from build123d import *

# Parameters (mm, degrees)
F0_R     = 5.5
F0_R_2   = 1
F1_DEPTH = 3
F2_R     = 5
F2_R_2   = 1
F3_DEPTH = 3
F4_W     = 8
F4_H     = 6
F4_R     = 1
F5_DEPTH = 8
F6_R     = 1
F7_DEPTH = 25


with BuildPart() as f1:
    # F0 (on Top) → F1 (new body)
    with BuildSketch(Plane.XY):
        with Locations((-27.4031814188, 27.8583839536)):
            Circle(F0_R)
        with Locations((-27.4031814188, 27.8583839536)):
            Circle(F0_R_2, mode=Mode.SUBTRACT)
    extrude(amount=F1_DEPTH)

    # F2 (on face) → F3 (join)
    with BuildSketch(Plane.XY.offset(3)):
        with Locations((-27.4031814188, 27.8583839536)):
            Circle(F2_R)
        with Locations((-27.4031814188, 27.8583839536)):
            Circle(F2_R_2, mode=Mode.SUBTRACT)
    extrude(amount=F3_DEPTH)

    # F4 (on face) → F5 (join)
    with BuildSketch(Plane.XY.offset(6)):
        with Locations((-27.4031814188, 27.8583839536)):
            Rectangle(F4_W, F4_H)
        with Locations((-27.4031814188, 27.8583839536)):
            Circle(F4_R, mode=Mode.SUBTRACT)
        with Locations((-27.4031814188, 27.8583839536)):
            Circle(F4_R)
    extrude(amount=F5_DEPTH)

    # F6 (on face) → F7 (cut)
    with BuildSketch(Plane.XZ.offset(-24.8583839536)):
        with Locations((-27.4031814188, 10)):
            Circle(F6_R)
    extrude(amount=-F7_DEPTH, mode=Mode.SUBTRACT)


solid = f1.part
Check sheet for the modelled part. Datum: model origin and axes. Units: mm. A direction names the side the tool comes from. Give positions to 0.01 mm unless a question says otherwise; leave off trailing zeros. Write each loop counter-clockwise with the first axis right and the second up, starting at its lowest first coordinate (ties: lowest second). Pieces come first, ordered by that corner, then holes. Notation, with made-up numbers: (69.25, 1.25) -> (73.25, 1.25) arc R32 cw to (73.25, 33.25) -> close; hole circle Ø10 at (-21.5, -2). An arc over 180 degrees is marked (long way). Write item = value, one per line.
Item 1: Gauge pin test, flat ends, axial feed: pin 1 (2 mm diameter, centred on x = -28.5, y = 32, fed in from +Z); pin 2 (3 mm diameter, centred on y = 25, z = 9.5, fed in from -X); pin 3 (0.6 mm diameter, centred on x = -27, y = 27.5, fed in from -Z); pin 4 (4 mm diameter, centred on x = -28.5, y = 26.5, fed in from -Z). Record the tip position at first contact, or that the pin passes through.
Output:
pin_1 = 6
pin_2 = -31.4
pin_3 = 6
pin_4 = 0
Item 2: Sectioned sample at B-B on x = -27.5. Record the boundary of the cut face in (y, z).
Output:
outline = (22.36, 0) -> (26.86, 0) -> (26.86, 6) -> (28.85, 6) -> (28.85, 0) -> (33.36, 0) -> (33.36, 3) -> (32.86, 3) -> (32.86, 6) -> (30.86, 6) -> (30.86, 9) -> (24.86, 9) -> (24.86, 6) -> (22.86, 6) -> (22.86, 3) -> (22.36, 3) -> close; (24.86, 11) -> (30.86, 11) -> (30.86, 14) -> (24.86, 14) -> close
Item 3: Sectioned sample at C-C on y = 28.25. Record the boundary of the cut face in (x, z), and give its area (3 significant figures).
Output:
outline = (-32.89, 0) -> (-28.32, 0) -> (-28.32, 6) -> (-26.48, 6) -> (-26.48, 0) -> (-21.92, 0) -> (-21.92, 3) -> (-22.42, 3) -> (-22.42, 6) -> (-23.4, 6) -> (-23.4, 14) -> (-31.4, 14) -> (-31.4, 6) -> (-32.39, 6) -> (-32.39, 3) -> (-32.89, 3) -> close; hole circle Ø2 at (-27.4, 10)
area = 113 mm^2
Item 4: Sectioned sample at D-D on x = -24.5. Record the boundary of the cut face in (y, z), and give its area (3 significant figures).
Output:
outline = (23.19, 0) -> (32.53, 0) -> (32.53, 3) -> (31.93, 3) -> (31.93, 6) -> (30.86, 6) -> (30.86, 14) -> (24.86, 14) -> (24.86, 6) -> (23.79, 6) -> (23.79, 3) -> (23.19, 3) -> close
area = 100 mm^2
Item 5: Scan lines: probe 1 along Z at (x, y) = (-27.75, 31); probe 2 along X at (y, z) = (28.75, 11.5); probe 3 along Y at (x, z) = (-28, 7). Record each from-to range of solid material in increasing order. Write a range as from..to.
Output:
probe_1 = 0..6
probe_2 = -31.4..-23.4
probe_3 = 24.86..30.86
Item 6: Tool access check on faces 4 (the flat face through (-27, 24, 6)), 5 (the flat face through (-26.6, 30.858, 9.1)), 6 (the cylindrical face through (-31.088, 31.238, 4.479)), 7 (the flat face through (-27, 28, 6)). Record the directions out of +Z, -Z, +X, -X, +Y, -Y that give a thin tool (end or side, any length) a straight path to the whole face; none if there is none.
Output:
face_4 = +Z, +X, -X, -Y
face_5 = +Z, +X, -X, +Y
face_6 = +Z
face_7 = -Z
Item 7: Release check for a two-part mould opening along X. For faces 1 (the cylindrical face through (-26.45, 27.82, 10.3)), 2 (the flat face through (-23.403, 28, 10)), 3 (the flat face through (-27, 32, 6)) record: +X half, -X half, draft (parallel to the pull), parting line (faces both ways), or undercut.
Output:
face_1 = undercut
face_2 = +X half
face_3 = draft
Item 8: Sectioned sample at A-A on z = 10. Record the boundary of the cut face in (x, y).
Output:
outline = (-31.4, 24.86) -> (-28.4, 24.86) -> (-28.4, 30.86) -> (-31.4, 30.86) -> close; (-26.4, 24.86) -> (-23.4, 24.86) -> (-23.4, 30.86) -> (-26.4, 30.86) -> close
